The model under review builds one solid part; all positions refer to its coordinate system, in mm. A direction names the side the tool comes from. Coordinates: 2 decimals unless noted, no trailing zeros. Write each loop counter-clockwise with the first axis right and the second up, starting at its lowest first coordinate (ties: lowest second). Pieces come first, ordered by that corner, then holes. Notation, with made-up numbers: (-17.75, -23.75) -> (19.25, -23.75) arc R35 cw to (19.25, 13.25) -> close; hole circle Ø4 at (66, 74). An arc over 180 degrees is marked (long way). Put each result on its own line as item: value. Start each with the question number.
from build123d import *

# Parameters (mm, degrees)
SKETCH1_R           = 2.5
BOSS_EXTRUDE1_DEPTH = 1.813873007
SKETCH2_R           = 1.5
CUT_EXTRUDE1_DEPTH  = 62.469831099


with BuildPart() as part:
    # Sketch1 → Boss-Extrude1 (new body)
    with BuildSketch(Plane.XY):
        with BuildLine():
            Line((36.25, -10), (36.25, 10))
            ThreePointArc((36.25, 10), (40.919052696, 17.33292647), (47.494545324, 23.019292657))
            ThreePointArc((47.494545324, 23.019292657), (49.358557668, 32.179111268), (40.140588391, 33.730195219))
            ThreePointArc((40.140588391, 33.730195219), (33.169485012, 29.243195432), (25.683959799, 25.68))
            ThreePointArc((25.683959799, 25.68), (21.013241966, 26.747299206), (18.027864045, 23))
            Line((18.027864045, 23), (-18.027864045, 23))
            ThreePointArc((-18.027864045, 23), (-21.013241966, 26.747299206), (-25.683959799, 25.68))
            ThreePointArc((-25.683959799, 25.68), (-33.169485012, 29.243195432), (-40.140588391, 33.730195219))
            ThreePointArc((-40.140588391, 33.730195219), (-49.358557668, 32.179111268), (-47.494545324, 23.019292657))
            ThreePointArc((-47.494545324, 23.019292657), (-40.919052696, 17.33292647), (-36.25, 10))
            Line((-36.25, 10), (-36.25, -10))
            ThreePointArc((-36.25, -10), (-40.919052696, -17.33292647), (-47.494545324, -23.019292657))
            ThreePointArc((-47.494545324, -23.019292657), (-49.358557668, -32.179111268), (-40.140588391, -33.730195219))
            ThreePointArc((-40.140588391, -33.730195219), (-33.169485012, -29.243195432), (-25.683959799, -25.68))
            ThreePointArc((-25.683959799, -25.68), (-21.013241966, -26.747299206), (-18.027864045, -23))
            Line((-18.027864045, -23), (18.027864045, -23))
            ThreePointArc((18.027864045, -23), (21.013241966, -26.747299206), (25.683959799, -25.68))
            ThreePointArc((25.683959799, -25.68), (33.169485012, -29.243195432), (40.140588391, -33.730195219))
            ThreePointArc((40.140588391, -33.730195219), (49.358557668, -32.179111268), (47.494545324, -23.019292657))
            ThreePointArc((47.494545324, -23.019292657), (40.919052696, -17.33292647), (36.25, -10))
        make_face()
        with Locations((-44, -28.5)):
            Circle(SKETCH1_R, mode=Mode.SUBTRACT)
        with Locations(Location((-44, 28.5, 0), (0, 0, 180))):
            Circle(SKETCH1_R, mode=Mode.SUBTRACT)
        with Locations(Location((44, -28.5, 0), (0, 0, 180))):
            Circle(SKETCH1_R, mode=Mode.SUBTRACT)
        with Locations((44, 28.5)):
            Circle(SKETCH1_R, mode=Mode.SUBTRACT)
    extrude(amount=BOSS_EXTRUDE1_DEPTH)

    # Sketch2 → Cut-Extrude1 (cut, through all)
    with BuildSketch(Plane.XY.offset(1.813873007)):
        with Locations((-22.5, 22.5)):
            Circle(SKETCH2_R)
        with Locations(Location((-22.5, -22.5, 0), (0, 0, 180))):
            Circle(SKETCH2_R)
        with Locations((22.5, -22.5)):
            Circle(SKETCH2_R)
        with Locations(Location((22.5, 22.5, 0), (0, 0, 180))):
            Circle(SKETCH2_R)
        with BuildLine():
            Line((-7.765, 16.5), (7.765, 16.5))
            ThreePointArc((7.765, 16.5), (8.68337839, 15.89570334), (8.491810792, 14.813162266))
            Line((8.491810792, 14.813162266), (0.726810792, 6.596249413))
            ThreePointArc((0.726810792, 6.596249413), (0, 6.283087147), (-0.726810792, 6.596249413))
            Line((-0.726810792, 6.596249413), (-8.491810792, 14.813162266))
            ThreePointArc((-8.491810792, 14.813162266), (-8.68337839, 15.89570334), (-7.765, 16.5))
        make_face()
        with BuildLine():
            Line((-7.765, -16.5), (7.765, -16.5))
            ThreePointArc((7.765, -16.5), (8.68337839, -15.89570334), (8.491810792, -14.813162266))
            Line((8.491810792, -14.813162266), (0.726810792, -6.596249413))
            ThreePointArc((0.726810792, -6.596249413), (0, -6.283087147), (-0.726810792, -6.596249413))
            Line((-0.726810792, -6.596249413), (-8.491810792, -14.813162266))
            ThreePointArc((-8.491810792, -14.813162266), (-8.68337839, -15.89570334), (-7.765, -16.5))
        make_face()
        with BuildLine():
            Line((-24, -7.765), (-24, 7.765))
            ThreePointArc((-24, 7.765), (-23.395885369, 8.683299937), (-22.31345045, 8.492083019))
            Line((-22.31345045, 8.492083019), (-14.090009559, 0.727083019))
            ThreePointArc((-14.090009559, 0.727083019), (-13.776559109, 0), (-14.090009559, -0.727083019))
            Line((-14.090009559, -0.727083019), (-22.31345045, -8.492083019))
            ThreePointArc((-22.31345045, -8.492083019), (-23.395885369, -8.683299937), (-24, -7.765))
        make_face()
        with BuildLine():
            Line((24, -7.765), (24, 7.765))
            ThreePointArc((24, 7.765), (23.395885369, 8.683299937), (22.31345045, 8.492083019))
            Line((22.31345045, 8.492083019), (14.090009559, 0.727083019))
            ThreePointArc((14.090009559, 0.727083019), (13.776559109, 0), (14.090009559, -0.727083019))
            Line((14.090009559, -0.727083019), (22.31345045, -8.492083019))
            ThreePointArc((22.31345045, -8.492083019), (23.395885369, -8.683299937), (24, -7.765))
        make_face()
    extrude(amount=-CUT_EXTRUDE1_DEPTH, mode=Mode.SUBTRACT)


solid = part.part
1. The part is to be moulded in two halves that separate along Y. For faces 4 (the flat face through (-1, 0, 0)), 5 (the cylindrical face through (21.08, 26.77, 0.89)), 6 (the flat face through (4.7, 10.8, 0.9)), say which applies: released by +Y, released by -Y, zero draft, split by the parting line, or undercut.
2. Consider section A-A on y = -28.5. State the section outline as (x, z) points, then the cut area to 3 significant figures.
3. Consider section C-C on z = 0.8. State how many separate pieces and enclosed holes the cut face has, then the cut area to 3 significant figures.
4. Consider section B-B on x = 44. State the section outline as (y, z) points.
5. Wall thickness on line 1 (Y direction, x = -44, z = 0.6); line 2 (Y direction, x = 42, z = 0.25); line 3 (X direction, y = -5.5, z = 1.6): over which ranges is each line inside the solid? List them lowest first. Write a range as from..to.
6. Tool access review of faces 1 (the flat face through (-4.555, 10.647, 0.92)), 2 (the cylindrical face through (-33.27, -29.3, 0.89)), 3 (the cylindrical face through (-40.84, -17.24, 0.89)): name each direction out of +Z, -Z, +X, -X, +Y, -Y from which nothing blocks a thin tool from reaching the whole face with its end or side.
7. Insertion check: P1, Ø0.9, axis at y = -1.5, z = 1.5, coming from the +X side; P2, Ø0.9, axis at y = -2.5, z = 0.5, coming from the -X side; P3, Ø0.9, axis at x = 3, z = 1, coming from the +Y side. Each pin has a flat end and moves straight along its axis. Give the tip position at first contact, or say it passes through.
8. Consider section D-D on x = -16. State the section outline as (y, z) points, then the cut area to 3 significant figures.
Output values:
1. face 4: zero draft
1. face 5: released by +Y
1. face 6: undercut
2. outline: (-50.5, 0) -> (-46.5, 0) -> (-46.5, 1.81) -> (-50.5, 1.81) -> close; (-41.5, 0) -> (-31.8, 0) -> (-31.8, 1.81) -> (-41.5, 1.81) -> close; (31.8, 0) -> (41.5, 0) -> (41.5, 1.81) -> (31.8, 1.81) -> close; (46.5, 0) -> (50.5, 0) -> (50.5, 1.81) -> (46.5, 1.81) -> close
2. area: 49.7 mm^2
3. separate pieces: 1
3. enclosed holes: 12
3. area: 3,940 mm^2
4. outline: (-35, 0) -> (-31, 0) -> (-31, 1.81) -> (-35, 1.81) -> close; (-26, 0) -> (-20.42, 0) -> (-20.42, 1.81) -> (-26, 1.81) -> close; (20.42, 0) -> (26, 0) -> (26, 1.81) -> (20.42, 1.81) -> close; (31, 0) -> (35, 0) -> (35, 1.81) -> (31, 1.81) -> close
5. line 1: y = -35..-31, -26..-20.42, 20.42..26, 31..35
5. line 2: y = -34.68..-30, -27..-18.52, 18.52..27, 30..34.68
5. line 3: x = -36.25..-24, -19.14..19.14, 24..36.25
6. face 1: +Z, -Z
6. face 2: +Z, -Z, -Y
6. face 3: +Z, -Z, -X
7. P1: stops at x = 36.25
7. P2: stops at x = -36.25
7. P3: stops at y = 23
8. outline: (-23, 0) -> (-2.53, 0) -> (-2.53, 1.81) -> (-23, 1.81) -> close; (2.53, 0) -> (23, 0) -> (23, 1.81) -> (2.53, 1.81) -> close
8. area: 74.3 mm^2
